The figure shows three views and two pictorial views of one solid part (mm, origin at its lowest corner). Answer the questions. A direction names the side the tool comes from. Give positions to 0.01 mm unless a question says otherwise; leave off trailing zeros. Loops run counter-clockwise (first coordinate to the right, second up) from the corner with the lowest first, then second, coordinate; pieces in that order, holes last. Notation, with made-up numbers: (-36.75, -24.75) - (-20.75, -24.75) arc R28 cw to (-20.75, 12.25) - close; hole circle Ø3 at (85, 24.5). An arc over 180 degrees is marked (long way). One line per question, with ' | ' between items.
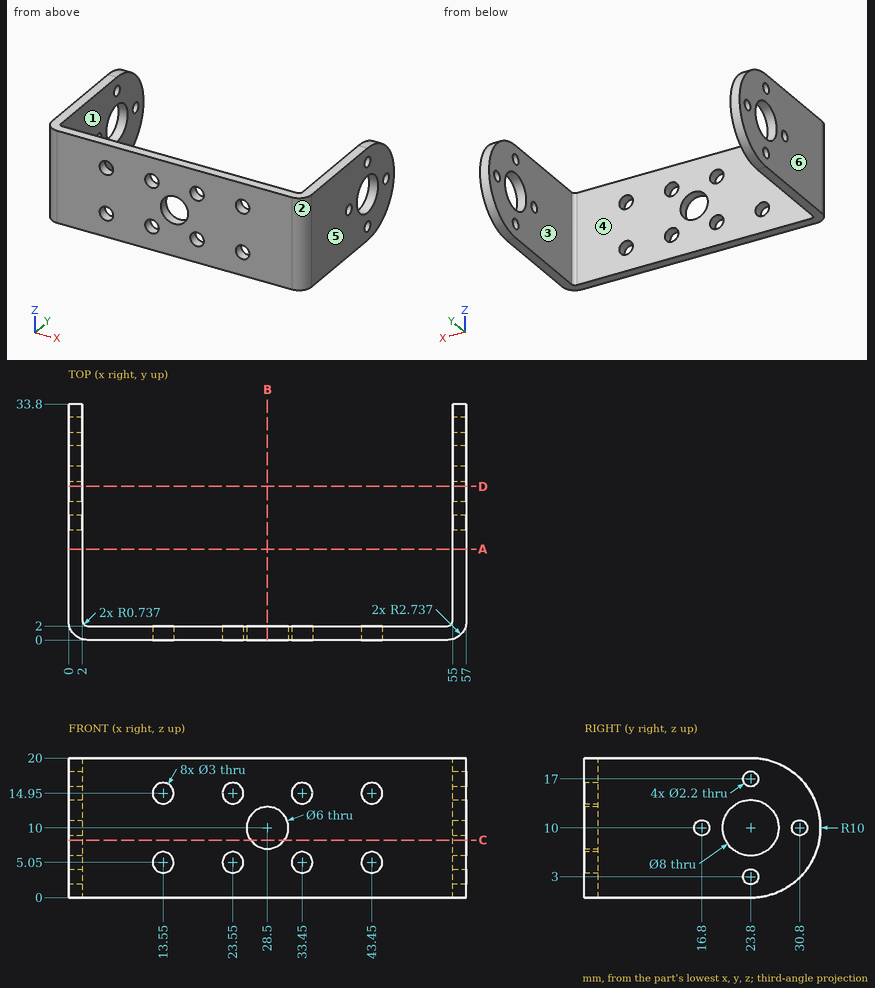
1. Flat-ended cylindrical pins translate along their axes: pin 1 (1.3 mm diameter, centred on y = 23.8, z = 17, fed in from +X) (1 decimal); pin 2 (3 mm diameter, centred on x = 20.5, z = 11, fed in from +Y). Find the tip coordinate at first contact, or state that the pin passes through.
Evaluation:
pin 1: through | pin 2: y = 2
2. Find section D-D on y = 22. Write down the section's boundary in (x, z).
Evaluation:
outline: (0, 0) - (2, 0) - (2, 6.43) - (0, 6.43) - close; (0, 13.57) - (2, 13.57) - (2, 20) - (0, 20) - close; (55, 0) - (57, 0) - (57, 6.43) - (55, 6.43) - close; (55, 13.57) - (57, 13.57) - (57, 20) - (55, 20) - close
3. Consider L1, parallel to Y at x = 55.8, z = 10; L2, parallel to X at y = 21, z = 6; L3, parallel to Y at x = 1.55, z = 10. Determine where each line is inside the solid, lowest interval first.
Evaluation:
L1: 0.47 to 15.7, 17.9 to 19.8, 27.8 to 29.7, 31.9 to 33.8 | L2: 0 to 2, 55 to 57 | L3: 0.27 to 15.7, 17.9 to 19.8, 27.8 to 29.7, 31.9 to 33.8
4. Find section B-B on x = 28.5. Write down the section's boundary in (y, z), then the cut area to 3 significant figures.
Evaluation:
outline: (0, 0) - (2, 0) - (2, 7) - (0, 7) - close; (0, 13) - (2, 13) - (2, 20) - (0, 20) - close | area: 28.0 mm2
5. Which of the six approach directions +Z, -Z, +X, -X, +Y, -Y give full straight-line access (tool end or side, diameter ignored) to the marked faces 1 and 2?
Evaluation:
face 1: +Z, -Z, +Y | face 2: +Z, -Z, +X, -Y
6. Find section A-A on y = 13. Write down the section's boundary in (x, z).
Evaluation:
outline: (0, 0) - (2, 0) - (2, 20) - (0, 20) - close; (55, 0) - (57, 0) - (57, 20) - (55, 20) - close
7. Determine the mould class of the marked faces 3, 4, 5 and 6 for opening direction X: +X half, -X half, draft (parallel to the pull), parting line (faces both ways), or undercut.
Evaluation:
face 3: undercut | face 4: undercut | face 5: +X half | face 6: -X half
8. Find section C-C on z = 8.25. Write down the section's boundary in (x, y) (1 decimal), then the cut area to 3 significant figures.
Evaluation:
outline: (0, 2.7) arc R2.7 ccw to (2.7, 0) - (26.1, 0) - (26.1, 2) - (2.7, 2) arc R0.7 cw to (2, 2.7) - (2, 20.2) - (0, 20.2) - close; (0, 27.4) - (2, 27.4) - (2, 33.6) - (0, 33.6) - close; (30.9, 0) - (54.3, 0) arc R2.7 ccw to (57, 2.7) - (57, 20.2) - (55, 20.2) - (55, 2.7) arc R0.7 cw to (54.3, 2) - (30.9, 2) - close; (55, 27.4) - (57, 27.4) - (57, 33.6) - (55, 33.6) - close | area: 199 mm2
